Verification items for the finished model (mm, model axes). Face numbers are marked on the shaded views. A direction names the side the tool comes from. Round coordinates to 2 decimals unless told otherwise and drop trailing zeros. Loops run counter-clockwise (first coordinate to the right, second up) from the corner with the lowest first, then second, coordinate; pieces in that order, holes last. Notation, with made-up numbers: M 76,23 L 129,23 A13 ccw 129,41 Z; hole C 88.25,-13.75 d11. An arc over 180 degrees is marked long. Write item = value, one per line. Start each with the question number.
from build123d import *

# Parameters (mm, degrees)
F1_DEPTH = 70
F2_R     = 12.5
F3_DEPTH = 20
F4_R     = 12.5
F5_DEPTH = 20
F7_DEPTH = 20
F9_DEPTH = 20


with BuildPart() as f1:
    # F0 (on Top) → F1 (new body)
    with BuildSketch(Plane.XY):
        Polygon((-7.5, 12.990381), (-15, 0), (-7.5, -12.990381), (7.5, -12.990381), (15, 0), (7.5, 12.990381), align=None)
    extrude(amount=F1_DEPTH)

    # F2 (on face) → F3 (join)
    with BuildSketch(Plane.XY.offset(70)):
        Circle(F2_R)
    extrude(amount=F3_DEPTH)

    # F4 (on face) → F5 (join)
    with BuildSketch(Plane(origin=(0, 0, 0), x_dir=(1, 0, 0), z_dir=(0, 0, -1))):
        Circle(F4_R)
    extrude(amount=F5_DEPTH)

    # F6 (on face) → F7 (join)
    with BuildSketch(Plane.XY.offset(90)):
        Polygon((5, 8.660254), (-5, 8.660254), (-10, 0), (-5, -8.660254), (5, -8.660254), (10, 0), align=None)
    extrude(amount=F7_DEPTH)

    # F8 (on face) → F9 (join)
    with BuildSketch(Plane(origin=(0, 0, -20), x_dir=(1, 0, 0), z_dir=(0, 0, -1))):
        Polygon((9.999949, 0.032092), (4.972181, 8.676256), (-5.027767, 8.644163), (-9.999949, -0.032092), (-4.972181, -8.676256), (5.027767, -8.644163), align=None)
    extrude(amount=F9_DEPTH)


solid = f1.part
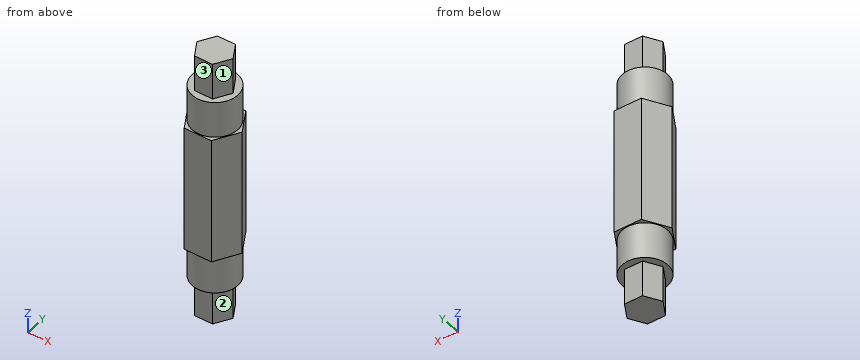
1. Section check C-C, the plane y = -5.75. Enter the section's corners in (x, z).
2. Tool access check on the marked faces 1, 2 and 3. Record the directions out of +Z, -Z, +X, -X, +Y, -Y that give a thin tool (end or side, any length) a straight path to the whole face; none if there is none.
3. Section check D-D, the plane z = 100. Enter the section's corners in (x, y), and give its area (3 significant figures).
4. Section check B-B, the plane x = 1.75. Enter the section's corners in (y, z).
5. Thickness scan on line 1 (X direction, y = 0.5, z = 74.5); line 2 (Y direction, x = -7.5, z = -12); line 3 (Y direction, x = 0.25, z = 80.5). Record the ranges inside material, lowest first.
6. Gauge pin test, flat ends, axial feed: P1, Ø8, axis at x = -1, z = 98.5, coming from the -Y side; P2, Ø10, axis at x = 7.5, y = -8, coming from the -Z side; P3, Ø2, axis at y = -2, z = 37, coming from the +X side; P4, Ø2, axis at y = 6.5, z = 31.5, coming from the +X side. Record the tip position at first contact, or that the pin passes through.
7. Section check A-A, the plane z = 2. Enter the section's corners in (x, y).
Computed values:
q1.outline = M -11.68,0 L -11.1,0 L -11.1,-20 L -6.69,-20 L -6.69,-40 L 6.67,-40 L 6.67,-20 L 11.1,-20 L 11.1,0 L 11.68,0 L 11.68,70 L 11.1,70 L 11.1,90 L 6.68,90 L 6.68,110 L -6.68,110 L -6.68,90 L -11.1,90 L -11.1,70 L -11.68,70 Z
q2.face_1 = +Z, +X, -Y
q2.face_2 = -Z, +X, -Y
q2.face_3 = +Z, +X, -X, -Y
q3.outline = M -10,0 L -5,-8.66 L 5,-8.66 L 10,0 L 5,8.66 L -5,8.66 Z
q3.area = 260 mm2
q4.outline = M -12.99,0 L -12.38,0 L -12.38,-20 L -8.67,-20 L -8.67,-40 L 8.65,-40 L 8.65,-20 L 12.38,-20 L 12.38,0 L 12.99,0 L 12.99,70 L 12.38,70 L 12.38,90 L 8.66,90 L 8.66,110 L -8.66,110 L -8.66,90 L -12.38,90 L -12.38,70 L -12.99,70 Z
q5.line_1 = -12.49 to 12.49
q5.line_2 = -10 to 10
q5.line_3 = -12.5 to 12.5
q6.P1 = -8.66
q6.P2 = -40
q6.P3 = 14.42
q6.P4 = 11.82
q7.outline = M -15,0 L -7.5,-12.99 L 7.5,-12.99 L 15,0 L 7.5,12.99 L -7.5,12.99 Z
